Design review of the part built by this model. Coordinates are the model's own, in mm. A direction names the side the tool comes from. Give positions to 0.01 mm unless a question says otherwise; leave off trailing zeros. Order: outer loops, then holes, each group sorted by start corner. A loop starts at its lowest first (then second) coordinate and runs counter-clockwise, first axis right, second up.
```python
from build123d import *

# Parameters (mm, degrees)
SKETCH2_R          = 27.5
CUT_EXTRUDE1_DEPTH = 260


with BuildPart() as part:
    # Sketch1 → Revolve1 (revolve)
    with BuildSketch(Plane.XY, mode=Mode.PRIVATE) as revolve1_sk:
        Polygon((-135, 95), (-135, 101), (0, 101), (0, 0), (-135, 0), (-135, 6), (-76.5, 6), (-76.5, 95), align=None)
    revolve(revolve1_sk.sketch.rotate(Axis((0, 0, 0), (0, 1, 0)), 270), axis=Axis((0, 0, 0), (0, 1, 0)))

    # Sketch2 → Cut-Extrude1 (cut)
    with BuildSketch(Plane(origin=(0, 101, 0), x_dir=(1, 0, 0), z_dir=(0, 1, 0))):
        with Locations(Location((0, 0, 0), (0, 0, 270))):
            Circle(SKETCH2_R)
    extrude(amount=-CUT_EXTRUDE1_DEPTH, mode=Mode.SUBTRACT)


solid = part.part
```
1. Take a section at A-A (x = 0). State the section outline as (y, z) points.
Recorded:
outline: (0, -135) - (6, -135) - (6, -76.5) - (95, -76.5) - (95, -135) - (101, -135) - (101, -27.5) - (0, -27.5) - close; (0, 27.5) - (101, 27.5) - (101, 135) - (95, 135) - (95, 76.5) - (6, 76.5) - (6, 135) - (0, 135) - close
2. Machinability: for faces 1 (the face through (119.77, 3.04, -62.29)), 2 (the face through (58, 95, 58)), which of the approach directions +Z, -Z, +X, -X, +Y, -Y give a long, thin tool a straight path to every point of the face, cutting with its end or side? Answer none if there is none.
Recorded:
face 1: +Y, -Y
face 2: none
3. For line 1 along X through (y, z) = (57, 0); line 2 along Y through (x, z) = (-37.5, -121.5); line 3 along X through (y, z) = (69, 8), list the stretches that pass through material, from the lowest coordinate up.
Recorded:
line 1: x = -76.5 to -27.5, 27.5 to 76.5
line 2: y = 0 to 6, 95 to 101
line 3: x = -76.08 to -26.31, 26.31 to 76.08
4. For pin 1 (3 mm diameter, centred on y = 34.5, z = -51, fed in from -X); pin 2 (6 mm diameter, centred on x = 28.5, y = 26.5, fed in from -Z); pin 3 (6 mm diameter, centred on x = -8, y = 86, fed in from -Z), all flat-tipped, find the tip position at first contact; note any pin that passes through.
Recorded:
pin 1: stops at x = -58.33
pin 2: stops at z = -72.12
pin 3: stops at z = -76.34
5. Take a section at B-B (z = 0). State the section outline as (x, y) points, then the cut area to 3 significant figures.
Recorded:
outline: (-135, 0) - (-27.5, 0) - (-27.5, 101) - (-135, 101) - (-135, 95) - (-76.5, 95) - (-76.5, 6) - (-135, 6) - close; (27.5, 0) - (135, 0) - (135, 6) - (76.5, 6) - (76.5, 95) - (135, 95) - (135, 101) - (27.5, 101) - close
area: 11,300 mm2
6. Take a section at D-D (y = 73). State the section outline as (x, z) points, then the cut area to 3 significant figures.
Recorded:
outline: circle Ø153 at (0, 0); hole circle Ø55 at (0, 0)
area: 16,000 mm2
7. Take a section at C-C (z = 33.5). State the section outline as (x, y) points (3 decimals).
Recorded:
outline: (-130.777, 0) - (130.777, 0) - (130.777, 6) - (68.775, 6) - (68.775, 95) - (130.777, 95) - (130.777, 101) - (-130.777, 101) - (-130.777, 95) - (-68.775, 95) - (-68.775, 6) - (-130.777, 6) - close
8. Draft analysis for pull direction Y (two halves, no side actions). For faces 3 (the face through (-24.397, 51.207, 12.69)), 4 (the face through (28, 101, 2)), 5 (the face through (74.68, 51.12, 16.58)), state which applies: pulls with the +Y half, pulls with the -Y half, needs draft (parallel to the pull), parting line crosses it, or undercut.
Recorded:
face 3: needs draft
face 4: pulls with the +Y half
face 5: undercut
